from build123d import *

# Parameters (mm, degrees)
F0_R     = 56.6775015073
F1_DEPTH = 101.6
F2_W     = 30.4712727666
F2_H     = 32.811390236
F3_DEPTH = 25.4
F4_W     = 9.221942164
F4_H     = 13.0037814379
F5_DEPTH = 73.66
F6_R     = 9.5030077165
F7_DEPTH = 50.8


with BuildPart() as f1:
    # F0 (on Top) → F1 (new body)
    with BuildSketch(Plane.XY):
        Circle(F0_R)
    extrude(amount=F1_DEPTH)

    # F2 (on face) → F3 (join)
    with BuildSketch(Plane.XY.offset(101.6)):
        with Locations((15.2356363833, 5.9477584437)):
            Rectangle(F2_W, F2_H)
    extrude(amount=F3_DEPTH)

    # F4 (on face) → F5 (join)
    with BuildSketch(Plane(origin=(0, 0, 0), x_dir=(0, -1, 0), z_dir=(-1, 0, 0))):
        with Locations((-13.5935484432, 113.1370440125)):
            Rectangle(F4_W, F4_H)
    extrude(amount=F5_DEPTH)

    # F6 (on face) → F7 (cut)
    with BuildSketch(Plane.XZ.offset(10.4579366744)):
        with Locations((14.3979880959, 114.1804158688)):
            Circle(F6_R)
    extrude(amount=-F7_DEPTH, mode=Mode.SUBTRACT)


solid = f1.part
Could you check a few things on this model? Use its own coordinates, in mm. A direction names the side the tool comes from. Give positions to 0.01 mm unless a question says otherwise; leave off trailing zeros. Order: outer loops, then holes, each group sorted by start corner. A loop starts at its lowest first (then second) coordinate and runs counter-clockwise, first axis right, second up. Notation, with made-up numbers: (85, 58.5) - (125, 58.5) arc R6 ccw to (125, 67.5) - close; hole circle Ø3 at (28, 58.5). An arc over 180 degrees is marked (long way). One line per question, with ' | ' between items. Start each with the question number.
Item 1: I want a section at A-A on x = -5.5. Write out the boundary of the cut face in (y, z).
Item 2: I want a section at D-D on x = -65.5. Write out the boundary of the cut face in (y, z), then the cut area to 3 significant figures.
Item 3: I'm going to push flat-ended pins straight in: pin 1 Ø3 at (x, z) = (32, 52.5) entering from +Y; pin 2 Ø6 at (y, z) = (-28.5, 81.5) entering from -X; pin 3 Ø1 at (x, y) = (-11, 35) entering from +Z; pin 4 Ø17 at (x, z) = (14.4, 114.18) entering from +Y. Where does each tip first touch, or does it pass through?
Item 4: I want a section at B-B on y = 0. Write out the boundary of the cut face in (x, z), then the cut area to 3 significant figures.
Item 5: I want a section at C-C on z = 87. Write out the boundary of the cut face in (x, y) (1 decimal), then the cut area to 3 significant figures.
Item 6: Thinking about a two-plate mould opening in Z: for faces 1 (the flat face through (15, 6, 127)), 2 (the cylindrical face through (12.338, 5.718, 104.903)), 3 (the flat face through (30.471, 6, 114)), which applies, pulls with the +Z half, pulls with the -Z half, needs draft (parallel to the pull), parting line crosses it, or undercut?
Item 7: I need wall thicknesses on probe 1 along Z at (x, y) = (15, -10); probe 2 along Z at (x, y) = (0.5, 27); probe 3 along X at (y, z) = (-6, 52.5). Which ranges of each line are inside material? Lowest first, please. Write a range as [from, to].
Item 8: For faces 4 (the flat face through (-36, 18.205, 113)), 5 (the flat face through (-36, 14, 119.639)), 6 (the flat face through (25, -10.458, 114)), which set-ups out of +Z, -Z, +X, -X, +Y, -Y let a thin tool reach every point of the face, with its end or its side?
Verdict:
1) outline: (-56.41, 0) - (56.41, 0) - (56.41, 101.6) - (-56.41, 101.6) - close; (8.98, 106.64) - (18.2, 106.64) - (18.2, 119.64) - (8.98, 119.64) - close
2) outline: (8.98, 106.64) - (18.2, 106.64) - (18.2, 119.64) - (8.98, 119.64) - close | area: 120 mm^2
3) pin 1: y = 47.77 | pin 2: x = -50.62 | pin 3: z = 101.6 | pin 4: through
4) outline: (-56.68, 0) - (56.68, 0) - (56.68, 101.6) - (30.47, 101.6) - (30.47, 127) - (0, 127) - (0, 101.6) - (-56.68, 101.6) - close; hole circle Ø19.01 at (14.4, 114.18) | area: 12,000 mm^2
5) outline: circle Ø113.4 at (0, 0) | area: 10,100 mm^2
6) face 1: pulls with the +Z half | face 2: undercut | face 3: needs draft
7) probe 1: [0, 104.7], [123.66, 127] | probe 2: [0, 101.6] | probe 3: [-56.36, 56.36]
8) face 4: +Z, -X, +Y | face 5: +Z, -X, +Y, -Y | face 6: +Z, +X, -X, -Y
